Read the model definition and answer for the solid it produces. Units are mm, in the model's axes. A direction names the side the tool comes from. Give positions to 0.01 mm unless a question says otherwise; leave off trailing zeros. Order: outer loops, then holes, each group sorted by start corner. A loop starts at its lowest first (then second) coordinate and runs counter-clockwise, first axis right, second up. Notation, with made-up numbers: M 25,87 L 50,87 A14 cw 50,91 Z; hole C 69,39 d1. An arc over 180 degrees is marked long. One line per item, written item: value.
Autodesk Inventor part; units mm, degrees
ref_plane "YZ Plane" through (0, 0, 0) normal (1, 0, 0) x (0, 1, 0)
ref_plane "XZ Plane" through (0, 0, 0) normal (0, 1, 0) x (-1, 0, 0)
ref_plane "XY Plane" through (0, 0, 0) normal (0, 0, 1) x (1, 0, 0)
sketch "Sketch1" plane through (0, 0, 0) normal (0, 1, 0) x (-1, 0, 0)
  line L0 (-15, 15.75) -> (-15, -15.75)
  line L1 (-15, -15.75) -> (15, -15.75)
  line L2 (15, -15.75) -> (15, 15.75)
  line L3 (15, 15.75) -> (-15, 15.75)
  line L4 (-15, 15.75) -> (15, -15.75) construction
  line L5 (-15, -15.75) -> (15, 15.75) construction
  point P0 (0, 0)
  dimension "d0" = 31.5
  dimension "d1" = 30
extrude "Extrusion1" add sketch "Sketch1" along normal blind 8
sketch "Sketch2" plane through (-15, 0, 15.75) normal (0, 0, 1) x (1, 0, 0)
  circle A0 centre (15, 4) radius 1.5
  line L0 (0, 8) -> (30, 8)
  point P0 (15, 0)
  dimension "d4" = 3
  dimension "d5" = 8
  dimension "d6" = 4
hole "Hole1" at (0, 4, 15.75) direction (0, 0, -1) diameter 3.88 depth 7 countersink diameter 4.34 countersink angle 7
pattern_linear "Rectangular Pattern1" count 2 spacing 10 along (1, 0, 0) count 2 spacing 10 along (-1, 0, 0) of "Hole1"
mirror "Mirror1" about plane through (0, 0, 0) normal (0, 0, 1) of "Hole1", "Rectangular Pattern1"
sketch "Sketch3" plane through (0, 0, 0) normal (0, -1, 0) x (1, 0, 0)
  line L0 (-15, -13) -> (-15, 13)
  line L1 (-15, 13) -> (15, 13)
  line L2 (15, 13) -> (15, -13)
  line L3 (15, -13) -> (-15, -13)
  line L4 (-15, -13) -> (15, 13) construction
  line L5 (-15, 13) -> (15, -13) construction
  point P0 (0, 0)
  dimension "d20" = 26
  dimension "d21" = 30
extrude "Extrusion2" add sketch "Sketch3" along normal blind 5
sketch "Sketch4" plane through (0, -5, 0) normal (0, -1, 0) x (1, 0, 0)
  circle A0 centre (0, 0) radius 40
  dimension "d24" = 80
extrude "Extrusion3" add sketch "Sketch4" along normal blind 6
fillet "Fillet1" radius 2 6 edges at (0, 0, 13) (0, -5, 13) (15, -5, 0) (0, -5, -13) (-15, -5, 0) (0, 0, -13)
properties part number "cycloid_fixing_base"
1) Each of these flat-tipped pins is pushed along its axis until it touches: pin 1 Ø1.1 at (x, y) = (-2.5, -2.5) entering from +Z; pin 2 Ø3 at (x, y) = (0, 4) entering from -Z; pin 3 Ø3 at (x, y) = (-10, 4) entering from +Z; pin 4 Ø2 at (y, z) = (-3, 18) entering from +X. Where does it stop, or does it pass through?
Reported:
pin 1: stops at z = 13
pin 2: stops at z = -8.75
pin 3: stops at z = 8.75
pin 4: passes through
2) Determine the mould class of faces 6 (the face through (15, 2, 0)), 7 (the face through (-8.69, 5.43, -10.35)), 8 (the face through (-15.6, -4.43, 0.21)), 9 (the face through (0, 8, 0)) for opening direction X: +X half, -X half, draft (parallel to the pull), parting line (faces both ways), or undercut.
Reported:
face 6: +X half
face 7: undercut
face 8: -X half
face 9: draft
3) Which of the six approach directions +Z, -Z, +X, -X, +Y, -Y give full straight-line access (tool end or side, diameter ignored) to faces 1 (the face through (15.6, -4.43, -0.21)), 2 (the face through (0, 4, 8.75)), 3 (the face through (-10, 4, -8.75)), 4 (the face through (0.21, -0.6, 13.57)), 5 (the face through (-15, 2, 0))?
Reported:
face 1: +Z, -Z, +X, +Y
face 2: +Z
face 3: -Z
face 4: +Z, +X, -X
face 5: +Z, -Z, -X, +Y
4) Find section C-C, the plane y = -6. Write down the section's boundary in (x, z), plus the area to 3 significant figures.
Reported:
outline: C 0,0 d80
area: 5,030 mm^2
5) Consider probe 1 along X at (y, z) = (4, -10.75); probe 2 along Y at (x, z) = (0, -9.8); probe 3 along X at (y, z) = (5.75, 15). Determine where each line is inside the solid, lowest interval first.
Reported:
probe 1: x = -15 to -11.94, -8.06 to -1.94, 1.94 to 8.06, 11.94 to 15
probe 2: y = -11 to 2.06, 5.94 to 8
probe 3: x = -15 to -11.2, -8.8 to -1.2, 1.2 to 8.8, 11.2 to 15
6) Find section B-B, the plane x = 0. Write down the section's boundary in (y, z), plus the area to 3 significant figures.
Reported:
outline: M -11,-40 L -5,-40 L -5,-15 A2 cw -3,-13 L -2,-13 A2 cw 0,-15 L 0,-15.75 L 1.83,-15.75 L 2.06,-11.99 L 2.06,-8.75 L 5.94,-8.75 L 5.94,-11.99 L 6.17,-15.75 L 8,-15.75 L 8,15.75 L 6.17,15.75 L 5.94,11.99 L 5.94,8.75 L 2.06,8.75 L 2.06,11.99 L 1.83,15.75 L 0,15.75 L 0,15 A2 cw -2,13 L -3,13 A2 cw -5,15 L -5,40 L -11,40 Z
area: 809 mm^2
7) Find section A-A, the plane z = 14. Write down the section's boundary in (x, y).
Reported:
outline: M -37.47,-11 L 37.47,-11 L 37.47,-5 L 17,-5 A2 cw 16,-4.73 L -16,-4.73 A2 cw -17,-5 L -37.47,-5 Z; M -15,-0.27 L 15,-0.27 L 15,8 L -15,8 Z; hole C -10,4 d4.13; hole C 0,4 d4.13; hole C 10,4 d4.13
8) Find section D-D, the plane z = -25.5. Write down the section's boundary in (x, y).
Reported:
outline: M -30.82,-11 L 30.82,-11 L 30.82,-5 L -30.82,-5 Z
